Work out the finished part from the listing and answer in its coordinate system (mm). A direction names the side the tool comes from. Give positions to 0.01 mm unless a question says otherwise; leave off trailing zeros. Write each loop counter-clockwise with the first axis right and the second up, starting at its lowest first coordinate (ties: lowest second). Pieces come first, ordered by that corner, then holes. Notation, with made-up numbers: (40, 40) -> (90, 40) arc R19 ccw to (90, 77) -> close; hole circle Ø5 at (54, -29.75). An arc over 180 degrees is marked (long way). Use a Markdown table: item, result. Add a question column.
Q1. For faces 5 (the face through (10, 40, 12)), 6 (the face through (-10, -40, 12)), 7 (the face through (32.502, 7.218, 12.325)), 8 (the face through (-30, 0, 12)), determine the directions among +Z, -Z, +X, -X, +Y, -Y from which every point of the face is accessible in a straight line to the end or side of a thin tool.
Q2. Section A-A, the plane y = -22 is taken. Give the vertices of the cut face in (x, z).
Q3. Section C-C, the plane y = 28.5 is taken. Give the vertices of the cut face in (x, z).
Q4. For a pull along X with two mould halves and no side action, classify faces 1 (the face through (-33, -27, 12)), 2 (the face through (27, -33, 12)), 3 (the face through (-21.084, -19.522, 24.65)), 4 (the face through (0, 30, 12)) as pulls with the +X half, pulls with the -X half, needs draft (parallel to the pull), parting line crosses it, or undercut.
Q5. Each of these flat-tipped pins is pushed along its axis until it touches: pin 1 Ø12 at (x, z) = (-11.5, 7.5) entering from -Y; pin 2 Ø6 at (x, y) = (-20, -14.64) entering from -Z; pin 3 Ø10 at (y, z) = (14, 12.5) entering from -X; pin 4 Ø10 at (x, z) = (34, 14.5) entering from -Y. Where does it stop, or does it pass through?
Q6. Section D-D, the plane x = 8.5 is taken. Give the vertices of the cut face in (y, z), plus the area to 3 significant figures.
Q7. Section B-B, the plane x = -26.5 is taken. Give the vertices of the cut face in (y, z), plus the area to 3 significant figures.
Q8. Consider line 1 (Y direction, x = -13.5, z = 33); line 2 (Y direction, x = -16.5, z = 44); line 3 (Y direction, x = -21, z = 12.5). Determine where each line is inside the solid, lowest interval first.
from build123d import *

# Parameters (mm, degrees)
F0_R     = 5
F1_DEPTH = 25
F2_DEPTH = 50


with BuildPart() as f1:
    # F0 (on Top) → F1 (new body)
    with BuildSketch(Plane.XY):
        Polygon((20, 0), (0, 0), (0, -20), (14.641016, -45.358984), (40, -20), (40, 0), align=None)
        with BuildLine():
            ThreePointArc((24.641016, -20), (22.572166, -26.09072), (17.221643, -29.661282))
            ThreePointArc((17.221643, -29.661282), (6.709867, -13.90928), (24.641016, -20))
        make_face(mode=Mode.SUBTRACT)
        with BuildLine():
            ThreePointArc((24.641016, -20), (6.709867, -13.90928), (17.221643, -29.661282))
            ThreePointArc((17.221643, -29.661282), (22.572166, -26.09072), (24.641016, -20))
        make_face()
        with Locations((14.641016, -20)):
            Circle(F0_R, mode=Mode.SUBTRACT)
        Polygon((0, -20), (0, 0), (-20, 0), (-45.358984, -14.641016), (-20, -40), (0, -40), align=None)
        with BuildLine():
            ThreePointArc((-10, -14.641016), (-18.69862, -24.555975), (-29.661282, -17.221643))
            ThreePointArc((-29.661282, -17.221643), (-21.30138, -4.726057), (-10, -14.641016))
        make_face(mode=Mode.SUBTRACT)
        with BuildLine():
            ThreePointArc((-10, -14.641016), (-21.30138, -4.726057), (-29.661282, -17.221643))
            ThreePointArc((-29.661282, -17.221643), (-18.69862, -24.555975), (-10, -14.641016))
        make_face()
        with Locations((-20, -14.641016)):
            Circle(F0_R, mode=Mode.SUBTRACT)
        Polygon((-20, 0), (0, 0), (0, 20), (-14.641016, 45.358984), (-40, 20), (-40, 0), align=None)
        with BuildLine():
            ThreePointArc((-4.641016, 20), (-20.731736, 12.068851), (-17.221643, 29.661282))
            ThreePointArc((-17.221643, 29.661282), (-8.550296, 27.931149), (-4.641016, 20))
        make_face(mode=Mode.SUBTRACT)
        with BuildLine():
            ThreePointArc((-4.641016, 20), (-8.550296, 27.931149), (-17.221643, 29.661282))
            ThreePointArc((-17.221643, 29.661282), (-20.731736, 12.068851), (-4.641016, 20))
        make_face()
        with Locations((-14.641016, 20)):
            Circle(F0_R, mode=Mode.SUBTRACT)
        with Locations((-14.641016, 20)):
            Circle(F0_R)
        Polygon((0, 20), (0, 0), (20, 0), (45.358984, 14.641016), (20, 40), (0, 40), align=None)
        with BuildLine():
            ThreePointArc((30, 14.641016), (10.085041, 13.339636), (29.661282, 17.221643))
            ThreePointArc((29.661282, 17.221643), (29.914959, 15.942396), (30, 14.641016))
        make_face(mode=Mode.SUBTRACT)
        with BuildLine():
            ThreePointArc((30, 14.641016), (29.914959, 15.942396), (29.661282, 17.221643))
            ThreePointArc((29.661282, 17.221643), (10.085041, 13.339636), (30, 14.641016))
        make_face()
        with Locations((20, 14.641016)):
            Circle(F0_R, mode=Mode.SUBTRACT)
    extrude(amount=F1_DEPTH)

    # F0 (on Top) → F2 (join)
    with BuildSketch(Plane.XY):
        with BuildLine():
            ThreePointArc((-4.641016, 20), (-8.550296, 27.931149), (-17.221643, 29.661282))
            ThreePointArc((-17.221643, 29.661282), (-20.731736, 12.068851), (-4.641016, 20))
        make_face()
        with Locations((-14.641016, 20)):
            Circle(F0_R, mode=Mode.SUBTRACT)
        with BuildLine():
            ThreePointArc((-10, -14.641016), (-21.30138, -4.726057), (-29.661282, -17.221643))
            ThreePointArc((-29.661282, -17.221643), (-18.69862, -24.555975), (-10, -14.641016))
        make_face()
        with Locations((-20, -14.641016)):
            Circle(F0_R, mode=Mode.SUBTRACT)
        with BuildLine():
            ThreePointArc((24.641016, -20), (6.709867, -13.90928), (17.221643, -29.661282))
            ThreePointArc((17.221643, -29.661282), (22.572166, -26.09072), (24.641016, -20))
        make_face()
        with Locations((14.641016, -20)):
            Circle(F0_R, mode=Mode.SUBTRACT)
        with BuildLine():
            ThreePointArc((30, 14.641016), (29.914959, 15.942396), (29.661282, 17.221643))
            ThreePointArc((29.661282, 17.221643), (10.085041, 13.339636), (30, 14.641016))
        make_face()
        with Locations((20, 14.641016)):
            Circle(F0_R, mode=Mode.SUBTRACT)
    extrude(amount=F2_DEPTH)


solid = f1.part
Result set:
| question | item | result |
|---|---|---|
| 1 | face 5 | +Z, -Z, +X, +Y |
| 1 | face 6 | +Z, -Z, -X, -Y |
| 1 | face 7 | +Z, -Z, +X |
| 1 | face 8 | +Z, -Z, -X |
| 2 | outline | (-38, 0) -> (0, 0) -> (0, 25) -> (-13.23, 25) -> (-13.23, 50) -> (-26.77, 50) -> (-26.77, 25) -> (-38, 25) -> close; (1.15, 0) -> (10.06, 0) -> (10.06, 50) -> (4.84, 50) -> (4.84, 25) -> (1.15, 25) -> close; (19.22, 0) -> (38, 0) -> (38, 25) -> (24.44, 25) -> (24.44, 50) -> (19.22, 50) -> close |
| 3 | outline | (-31.5, 0) -> (-4.91, 0) -> (-4.91, 25) -> (-9.37, 25) -> (-9.37, 50) -> (-19.91, 50) -> (-19.91, 25) -> (-31.5, 25) -> close; (0, 0) -> (31.5, 0) -> (31.5, 25) -> (0, 25) -> close |
| 4 | face 1 | pulls with the -X half |
| 4 | face 2 | pulls with the +X half |
| 4 | face 3 | undercut |
| 4 | face 4 | undercut |
| 5 | pin 1 | stops at y = -40 |
| 5 | pin 2 | passes through |
| 5 | pin 3 | stops at x = -40 |
| 5 | pin 4 | stops at y = -31 |
| 6 | outline | (-34.72, 0) -> (40, 0) -> (40, 25) -> (-12.11, 25) -> (-12.11, 50) -> (-27.89, 50) -> (-27.89, 25) -> (-34.72, 25) -> close |
| 6 | area | 2,260 mm2 |
| 7 | outline | (-33.5, 0) -> (-3.75, 0) -> (-3.75, 25) -> (-7.04, 25) -> (-7.04, 50) -> (-22.24, 50) -> (-22.24, 25) -> (-33.5, 25) -> close; (0, 0) -> (33.5, 0) -> (33.5, 25) -> (0, 25) -> close |
| 7 | area | 1,960 mm2 |
| 8 | line 1 | y = -22.24 to -7.04, 10.07 to 15.13, 24.87 to 29.93 |
| 8 | line 2 | y = -24.01 to -18.21, -11.07 to -5.27, 10.17 to 15.36, 24.64 to 29.83 |
| 8 | line 3 | y = -39 to -19.54, -9.74 to -0.58, 0 to 39 |
